from build123d import *

# Parameters (mm, degrees)
SKETCH1_W           = 35.636
SKETCH1_H           = 55.178
BOSS_EXTRUDE1_DEPTH = 2
SKETCH2_W           = 3.23086443
SKETCH2_H           = 7.239
BOSS_EXTRUDE2_DEPTH = 19.685
SKETCH3_R           = 2.2225
CUT_EXTRUDE1_DEPTH  = 51.598920687
BOSS_EXTRUDE4_DEPTH = 1
BOSS_EXTRUDE5_DEPTH = 1


with BuildPart() as part:
    # Sketch1 → Boss-Extrude1 (new, symmetric)
    with BuildSketch(Plane.XY):
        with Locations((2.511331614, 1.04816211)):
            Rectangle(SKETCH1_W, SKETCH1_H)
    extrude(amount=BOSS_EXTRUDE1_DEPTH, both=True)

    # Sketch2 → Boss-Extrude2 (add)
    with BuildSketch(Plane.XY.offset(2)):
        with Locations((-13.691236171, 25.01766211)):
            Rectangle(SKETCH2_W, SKETCH2_H)
        with Locations((-13.691236171, -22.92133789)):
            Rectangle(SKETCH2_W, SKETCH2_H)
    extrude(amount=BOSS_EXTRUDE2_DEPTH)

    # Sketch3 → Cut-Extrude1 (cut, through all)
    with BuildSketch(Plane.ZY.offset(15.306668386)):
        with Locations(Location((16.9225, 26.09716211, 0), (0, 0, 270))):
            Circle(SKETCH3_R)
        with Locations(Location((16.9225, -24.00083789, 0), (0, 0, 270))):
            Circle(SKETCH3_R)
        with Locations(Location((6.7625, 26.09716211, 0), (0, 0, 270))):
            Circle(SKETCH3_R)
        with Locations(Location((6.7625, -24.00083789, 0), (0, 0, 270))):
            Circle(SKETCH3_R)
    extrude(amount=-CUT_EXTRUDE1_DEPTH, mode=Mode.SUBTRACT)

    # Sketch5 → Boss-Extrude4 (add)
    with BuildSketch(Plane.XZ.offset(26.54083789)):
        Polygon((-15.306668386, -2), (20.329331614, -2), (20.329331614, 2), (-12.075803956, 2), (-12.075803956, 21.685), (-15.306668386, 21.685), align=None)
    extrude(amount=BOSS_EXTRUDE4_DEPTH)

    # Sketch6 → Boss-Extrude5 (add)
    with BuildSketch(Plane(origin=(0, 28.63716211, 0), x_dir=(1, 0, 0), z_dir=(0, 1, 0))):
        Polygon((20.329331614, 2), (-15.306668386, 2), (-15.306668386, -21.685), (-12.075803956, -21.685), (-12.075803956, -2), (20.329331614, -2), align=None)
    extrude(amount=BOSS_EXTRUDE5_DEPTH)


solid = part.part
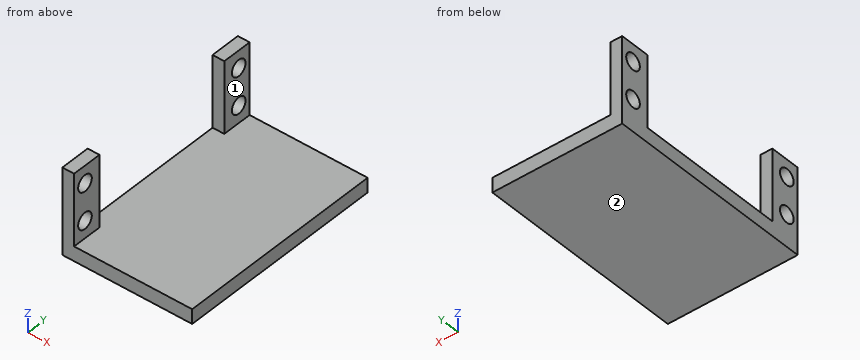
Can you work these out from the model? Positions are in its coordinate system, mm. Face numbers are marked on the shaded views. A direction names the side the tool comes from. Coordinates: 2 decimals unless noted, no trailing zeros. Write each loop counter-clockwise with the first axis right and the second up, starting at its lowest first coordinate (ties: lowest second). Pieces come first, ordered by that corner, then holes.
Q1. Imagine slicing it at C-C, the plane y = -1. List the corners of the cut face in (x, z) for me, plus the area to 3 significant figures.
Results found:
outline: (-15.31, -2) - (20.33, -2) - (20.33, 2) - (-15.31, 2) - close
area: 143 mm2
Q2. Imagine slicing it at D-D, the plane x = 9. List the corners of the cut face in (y, z) for me.
Results found:
outline: (-27.54, -2) - (29.64, -2) - (29.64, 2) - (-27.54, 2) - close
Q3. For P1, Ø1, axis at x = 12.5, y = 2.5, coming from the +Z side; P2, Ø9, axis at y = -23, z = 15, coming from the +X side, each with a flat end and sliding along its axis, tell me the tip position at first contact or that it passes through.
Results found:
P1: stops at z = 2
P2: stops at x = -12.08
Q4. Imagine slicing it at A-A, the plane z = 2.75. List the corners of the cut face in (x, y) for me.
Results found:
outline: (-15.31, -27.54) - (-12.08, -27.54) - (-12.08, -19.3) - (-15.31, -19.3) - close; (-15.31, 21.4) - (-12.08, 21.4) - (-12.08, 29.64) - (-15.31, 29.64) - close
Q5. Which directions (+Z, -Z, +X, -X, +Y, -Y) give clear straight access to the entire face, cutting with the end or side of a thin tool? Please do the marked faces 1 and 2.
Results found:
face 1: +Z, +X, +Y, -Y
face 2: -Z, +X, -X, +Y, -Y
Q6. Please list where these lines run through material, in increasing order: L1, parallel to X at y = -21, z = 20.5; L2, parallel to Z at x = 5, y = 4.5.
Results found:
L1: x = -15.31 to -12.08
L2: z = -2 to 2
Q7. Imagine slicing it at B-B, the plane z = 17.5. List the corners of the cut face in (x, y) for me.
Results found:
outline: (-15.31, -27.54) - (-12.08, -27.54) - (-12.08, -26.15) - (-15.31, -26.15) - close; (-15.31, -21.85) - (-12.08, -21.85) - (-12.08, -19.3) - (-15.31, -19.3) - close; (-15.31, 21.4) - (-12.08, 21.4) - (-12.08, 23.95) - (-15.31, 23.95) - close; (-15.31, 28.24) - (-12.08, 28.24) - (-12.08, 29.64) - (-15.31, 29.64) - close
